Verification items for the finished model (mm, model axes). Face numbers are marked on the shaded views. Coordinates: 2 decimals unless noted, no trailing zeros. Order: outer loops, then holes, each group sorted by start corner. A loop starts at its lowest first (then second) coordinate and runs counter-clockwise, first axis right, second up. Notation, with made-up numbers: (6, 11.25) - (14, 11.25) arc R15 ccw to (14, 28.25) - close; hole circle Ø4 at (53.5, 10.25). An arc over 180 degrees is marked (long way). Answer as CSV lines item,"result". Start each with the question number.
1. Section check C-C (z = 5.5). Record the cut outline in (x, y).
2. Go/stop test with flat-tipped pins: pin 1 (2 mm diameter, centred on x = 9, z = 2.5, fed in from -Y); pin 2 (3 mm diameter, centred on y = -4.5, z = 2, fed in from +X); pin 3 (1.5 mm diameter, centred on x = 17.5, z = 8.5, fed in from -Y). Record where each tip stops, or that it passes through.
3. Material ranges on L1, parallel to Y at x = 3, z = 9.25; L2, parallel to Y at x = 5, z = 1.25; L3, parallel to Y at x = 7.5, z = 9.5, recorded low to high. Write a range as [from, to].
4. Section check B-B (y = 0). Record the cut outline in (x, z).
5. Section check D-D (x = 31). Record the cut outline in (y, z), and give its area (3 significant figures).
6. Mould release check, pull along Y, two halves, no side actions. Record for the marked faces 1, 2 and 3: pulls with the +Y half, pulls with the -Y half, needs draft (parallel to the pull), parting line crosses it, or undercut.
7. Section check A-A (x = 19). Record the cut outline in (y, z).
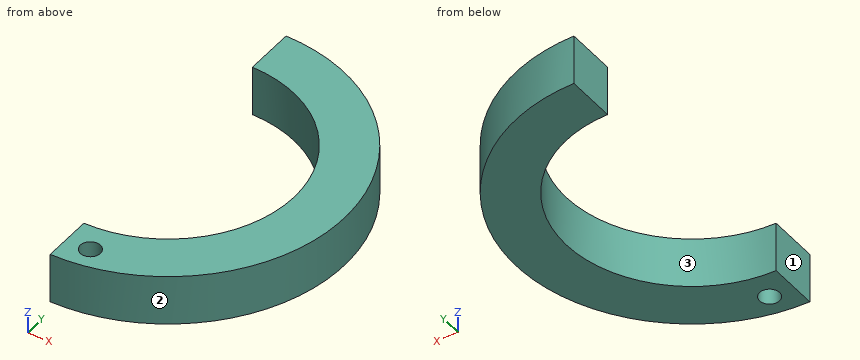
Autodesk Inventor part; units mm, degrees
ref_plane "YZ Plane" through (0, 0, 0) normal (1, 0, 0) x (0, 1, 0)
ref_plane "XZ Plane" through (0, 0, 0) normal (0, 1, 0) x (-1, 0, 0)
ref_plane "XY Plane" through (0, 0, 0) normal (0, 0, 1) x (1, 0, 0)
sketch "Sketch1" plane through (0, 0, 0) normal (0, 0, 1) x (1, 0, 0)
  circle A0 centre (0, 0) radius 35
  dimension "d0" = 70
extrude "Extrusion1" add sketch "Sketch1" along normal blind 10
sketch "Sketch2" plane through (0, 0, 10) normal (0, 0, 1) x (1, 0, 0)
  circle A0 centre (0, 0) radius 25
  line L0 (0, 34.925) -> (0, 25)
  line L1 (0, -25) -> (0, -34.925)
  line L2 (0, -30.1625) -> (4.7625, -30.1625)
  circle A1 centre (4.7625, -30.1625) radius 2
  dimension "d3" = 50
  dimension "d4" = 4
extrude "Extrusion2" cut sketch "Sketch2" against normal blind 10
sketch "Sketch3" plane through (0, 0, 10) normal (0, 0, 1) x (1, 0, 0)
  circle A0 centre (0, 0) radius 35
  line L0 (0, 35) -> (0, -35)
extrude "Extrusion3" cut sketch "Sketch3" against normal blind 10 contours L0 A0 picked at (-19.0322, -1.7332)
properties part number "5"
Evaluation:
1,outline,"(0, -35) arc R35 ccw to (0, 35) - (0, 25) arc R25 cw to (0, -25) - close; hole circle Ø4 at (4.76, -30.16)"
2,pin 1,"stops at y = -34.07"
2,pin 2,"stops at x = 34.87"
2,pin 3,"stops at y = -30.73"
3,L1,"y = [-34.87, -31.11], [-29.22, -24.82], [24.82, 34.87]"
3,L2,"y = [-34.64, -32.15], [-28.18, -24.49], [24.49, 34.64]"
3,L3,"y = [-34.19, -23.85], [23.85, 34.19]"
4,outline,"(25, 0) - (35, 0) - (35, 10) - (25, 10) - close"
5,outline,"(-16.25, 0) - (16.25, 0) - (16.25, 10) - (-16.25, 10) - close"
5,area,"325 mm²"
6,face 1,"needs draft"
6,face 2,"parting line crosses it"
6,face 3,"undercut"
7,outline,"(-29.39, 0) - (-16.25, 0) - (-16.25, 10) - (-29.39, 10) - close; (16.25, 0) - (29.39, 0) - (29.39, 10) - (16.25, 10) - close"
